Verification items for the finished model (mm, model axes). Round coordinates to 2 decimals unless told otherwise and drop trailing zeros. Write each loop counter-clockwise with the first axis right and the second up, starting at its lowest first coordinate (ties: lowest second). Pieces come first, ordered by that corner, then holes. Notation, with made-up numbers: M 35,51 L 59,51 A12 ccw 59,61 Z; hole C 27,1.5 d8. An arc over 180 degrees is marked long. One line per item, written item: value. Start each with the question number.
Item 1: Section check B-B, the plane y = -1.8. Record the cut outline in (x, z), then the cut area to 3 significant figures.
Item 2: Thickness scan on probe 1 along X at (y, z) = (-1.45, -41); probe 2 along Z at (x, y) = (38.5, -1.5). Record the ranges inside material, lowest first. Write a range as from..to.
Item 3: Section check A-A, the plane x = -48.5. Record the cut outline in (y, z) (3 decimals).
Item 4: Section check C-C, the plane z = -5.5. Record the cut outline in (x, y) (3 decimals).
from build123d import *

# Parameters (mm, degrees)
F0_W     = 134
F0_H     = 102
F1_DEPTH = 3.125
F2_W     = 29.5
F2_H     = 79.6
F3_DEPTH = 3.175
F5_W     = 29.5
F5_H     = 4.7
F6_DEPTH = 3.175


with BuildPart() as f1:
    # F0 (on Front) → F1 (new body)
    with BuildSketch(Plane.XZ):
        Rectangle(F0_W, F0_H)
    extrude(amount=F1_DEPTH)

    # F2 (on face) → F3 (cut)
    with BuildSketch(Plane.XZ.offset(3.125)):
        with Locations((-40.75, 0)):
            Rectangle(F2_W, F2_H)
        with Locations((38.25, 0)):
            Rectangle(F2_W, F2_H)
        with Locations((-1.25, 0)):
            Rectangle(F2_W, F2_H)
    extrude(amount=-F3_DEPTH, mode=Mode.SUBTRACT)

    # F5 (on face) → F6 (cut)
    with BuildSketch(Plane.XZ.offset(3.125)):
        with Locations((-40.75, 42.15)):
            Rectangle(F5_W, F5_H)
        with Locations((-1.25, 42.15)):
            Rectangle(F5_W, F5_H)
        with Locations((38.25, 42.15)):
            Rectangle(F5_W, F5_H)
        with Locations((38.25, -42.15)):
            Rectangle(F5_W, F5_H)
        with Locations((-1.25, -42.15)):
            Rectangle(F5_W, F5_H)
        with Locations((-40.75, -42.15)):
            Rectangle(F5_W, F5_H)
    extrude(amount=-F6_DEPTH, mode=Mode.SUBTRACT)


solid = f1.part
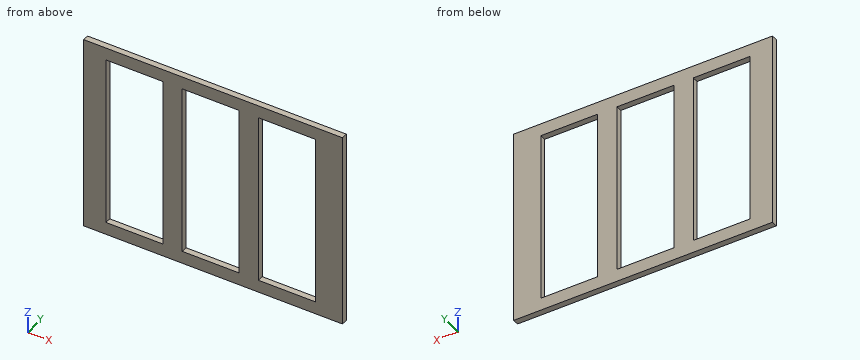
Response values:
1. outline: M -67,-51 L 67,-51 L 67,51 L -67,51 Z; hole M -55.5,-44.5 L -26,-44.5 L -26,44.5 L -55.5,44.5 Z; hole M -16,-44.5 L 13.5,-44.5 L 13.5,44.5 L -16,44.5 Z; hole M 23.5,-44.5 L 53,-44.5 L 53,44.5 L 23.5,44.5 Z
1. area: 5,790 mm2
2. probe 1: x = -67..-55.5, -26..-16, 13.5..23.5, 53..67
2. probe 2: z = -51..-44.5, 44.5..51
3. outline: M -3.125,-51 L 0,-51 L 0,-44.5 L -3.125,-44.5 Z; M -3.125,44.5 L 0,44.5 L 0,51 L -3.125,51 Z
4. outline: M -67,-3.125 L -55.5,-3.125 L -55.5,0 L -67,0 Z; M -26,-3.125 L -16,-3.125 L -16,0 L -26,0 Z; M 13.5,-3.125 L 23.5,-3.125 L 23.5,0 L 13.5,0 Z; M 53,-3.125 L 67,-3.125 L 67,0 L 53,0 Z
